Autodesk Inventor part; units mm, degrees
ref_plane "YZ Plane" through (0, 0, 0) normal (1, 0, 0) x (0, 1, 0)
ref_plane "XZ Plane" through (0, 0, 0) normal (0, 1, 0) x (-1, 0, 0)
ref_plane "XY Plane" through (0, 0, 0) normal (0, 0, 1) x (1, 0, 0)
sketch "草图1" plane through (0, 0, 0) normal (0, 0, 1) x (1, 0, 0)
  line L0 (0, 0) -> (0, 45) construction
  arc A0 (7.7977, 44.3192) -> (0, 45) centre (0, 0) ccw
  line L1 (0, 0) -> (13.1567, 43.0337) construction
  line L2 (0, 0) -> (0, 45) construction
  arc A1 (32.563, -44.3244) -> (32.563, 44.3244) centre (0, 0) ccw
  line L3 (0, 0) -> (16.0804, -52.5968) construction
  line L4 (0, 0) -> (16.0804, 52.5968) construction
  arc A2 (0, -45) -> (7.7977, -44.3192) centre (0, 0) ccw
  arc A3 (0, 45) -> (-7.7977, 44.3192) centre (0, 0) ccw
  arc A4 (-7.7977, -44.3192) -> (0, -45) centre (0, 0) ccw
  line L5 (0, 0) -> (45, 0) construction
  arc A5 (7.7977, 44.3192) -> (18.5563, 44.729) centre (12.2262, 69.489) ccw
  arc A6 (32.563, 44.3244) -> (23.7003, 46.0441) centre (26.3144, 35.8188) ccw
  line L6 (18.5563, 44.729) -> (23.7003, 46.0441)
  arc A7 (18.5563, -44.729) -> (7.7977, -44.3192) centre (12.2262, -69.489) ccw
  arc A8 (23.7003, -46.0441) -> (32.563, -44.3244) centre (26.3144, -35.8188) ccw
  line L7 (18.5563, -44.729) -> (23.7003, -46.0441)
  line L8 (0, 0) -> (-13.1567, 43.0337) construction
  line L9 (0, 0) -> (-13.1567, -43.0337) construction
  arc A9 (-25.925, 23.5137) -> (-25.925, -23.5137) centre (0, 0) ccw
  arc A10 (-7.7977, 44.3192) -> (-16.3105, 38.3374) centre (-5.674, 32.2489) ccw
  arc A11 (-25.925, 23.5137) -> (-20.6001, 30.8435) centre (-56.9437, 51.6471) ccw
  line L10 (-16.3105, 38.3374) -> (-20.6001, 30.8435)
  arc A12 (-16.3105, -38.3374) -> (-7.7977, -44.3192) centre (-5.674, -32.2489) ccw
  arc A13 (-20.6001, -30.8435) -> (-25.925, -23.5137) centre (-56.9437, -51.6471) ccw
  line L11 (-16.3105, -38.3374) -> (-20.6001, -30.8435)
  arc A14 (-7.7977, -44.3192) -> (7.7977, -44.3192) centre (0, 0) ccw construction
  arc A15 (13.1567, -43.0337) -> (-13.1567, -43.0337) centre (0, 0) ccw construction
  circle A16 centre (0, 0) radius 5
  dimension "d43" = 17
  dimension "d45" = 55
  dimension "d46" = 146
  dimension "d49" = 25.5563
  dimension "d50" = 5.3094
  dimension "d51" = 10.5541
  dimension "d52" = 17
  dimension "d53" = 34
  dimension "d54" = 35
  dimension "d55" = 12.2558
  dimension "d56" = 8.6348
  dimension "d57" = 41.8766
  dimension "凸轮孔直径" = 10
extrude "拉伸3" add sketch "草图1" along normal mid plane 15
properties part number "重要"
The model under review builds one solid part; all positions refer to its coordinate system, in mm. A direction names the side the tool comes from. Give positions to 0.01 mm unless a question says otherwise; leave off trailing zeros. Write each loop counter-clockwise with the first axis right and the second up, starting at its lowest first coordinate (ties: lowest second). Pieces come first, ordered by that corner, then holes. Notation, with made-up numbers: M -30,22.5 L 2,22.5 A28 ccw 2,52.5 Z; hole C 65.5,73 d5. An arc over 180 degrees is marked long. Answer in a Markdown table with one row per item.
Item 1: For line 1 along Y through (x, z) = (0, -3.25); line 2 along X through (y, z) = (2, -6.25); line 3 along Y through (x, z) = (-3.5, 5.25), list the stretches that pass through material, from the lowest coordinate up.
Check sheet entries:
| item | result |
|---|---|
| line 1 | -45 to -5, 5 to 45 |
| line 2 | -34.94 to -4.58, 4.58 to 54.96 |
| line 3 | -44.86 to -3.57, 3.57 to 44.86 |
Item 2: Tool access review of faces 1 (the face through (-18.425, -34.643, -0.105)), 2 (the face through (3.968, -44.825, -0.105)), 3 (the face through (21.092, 45.377, -0.105)): name each direction out of +Z, -Z, +X, -X, +Y, -Y from which nothing blocks a thin tool from reaching the whole face with its end or side.
Check sheet entries:
| item | result |
|---|---|
| face 1 | +Z, -Z, -X, -Y |
| face 2 | +Z, -Z, -Y |
| face 3 | +Z, -Z, +Y |
Item 3: Add section B-B on z = -3.25. Give the boundary of the cut face in (x, y) (1 decimal).
Check sheet entries:
| item | result |
|---|---|
| outline | M -25.9,-23.5 A41.9 cw -20.6,-30.8 L -16.3,-38.3 A12.3 ccw -7.8,-44.3 A45 ccw 0,-45 A45 ccw 7.8,-44.3 A25.6 cw 18.6,-44.7 L 23.7,-46 A10.6 ccw 32.6,-44.3 A55 ccw 32.6,44.3 A10.6 ccw 23.7,46 L 18.6,44.7 A25.6 cw 7.8,44.3 A45 ccw 0,45 A45 ccw -7.8,44.3 A12.3 ccw -16.3,38.3 L -20.6,30.8 A41.9 cw -25.9,23.5 A35 ccw Z; hole C 0,0 d10 |
Item 4: Add section A-A on y = 0. Give the boundary of the cut face in (x, z), plus the area to 3 significant figures.
Check sheet entries:
| item | result |
|---|---|
| outline | M -35,-7.5 L -5,-7.5 L -5,7.5 L -35,7.5 Z; M 5,-7.5 L 55,-7.5 L 55,7.5 L 5,7.5 Z |
| area | 1,200 mm2 |
Item 5: Add section C-C on y = -34. Give the boundary of the cut face in (x, z), plus the area to 3 significant figures.
Check sheet entries:
| item | result |
|---|---|
| outline | M -18.79,-7.5 L 43.23,-7.5 L 43.23,7.5 L -18.79,7.5 Z |
| area | 930 mm2 |
Item 6: Draft analysis for pull direction X (two halves, no side actions). For faces 4 (the face through (3.859, 44.834, -0.105)), 5 (the face through (9, 1, -7.5)), 6 (the face through (-12.66, -42.32, -0.11)), 7 (the face through (54.995, 0.722, -0.105)), state which applies: +X half, -X half, draft (parallel to the pull), parting line (faces both ways), or undercut.
Check sheet entries:
| item | result |
|---|---|
| face 4 | undercut |
| face 5 | draft |
| face 6 | -X half |
| face 7 | +X half |
Item 7: For P1, Ø6, axis at x = -19, z = -1, coming from the +Y side; P2, Ø5, axis at x = -14, z = 1, coming from the +Y side; P3, Ø2, axis at x = 45.5, z = -3, coming from the -Y side, all flat-tipped, find the tip position at first contact; note any pin that passes through.
Check sheet entries:
| item | result |
|---|---|
| P1 | y = 38.85 |
| P2 | y = 43.03 |
| P3 | y = -32.32 |
Item 8: Add section D-D on x = 40. Give the boundary of the cut face in (y, z), plus the area to 3 significant figures.
Check sheet entries:
| item | result |
|---|---|
| outline | M -37.75,-7.5 L 37.75,-7.5 L 37.75,7.5 L -37.75,7.5 Z |
| area | 1,130 mm2 |
